```python
from build123d import *

# Parameters (mm, degrees)
BOSS_EXTRUDE1_DEPTH                               = 450
BACKSIDEHOLES_SKETCH3_R                           = 1.5875
BACKSIDEHOLES_CUT_EXTRUDE1_DEPTH                  = 3.175
RIGHTSIDEHOLES_CUT_EXTRUDE2_OUTLINE_R             = 1.5875
RIGHTSIDEHOLES_CUT_EXTRUDE2_DEPTH                 = 3.175
CSK_FOR_6_FLAT_HEAD_MACHINE_SCREW_100_D           = 3.7973
CSK_FOR_6_FLAT_HEAD_MACHINE_SCREW_100_CSINK_D     = 7.0866
CSK_FOR_6_FLAT_HEAD_MACHINE_SCREW_100_CSINK_ANGLE = 100
CSK_FOR_6_FLAT_HEAD_MACHINE_SCREW_2_D             = 3.7973
CSK_FOR_6_FLAT_HEAD_MACHINE_SCREW_2_CSINK_D       = 7.0866
CSK_FOR_6_FLAT_HEAD_MACHINE_SCREW_2_CSINK_ANGLE   = 100


# Read off the part's stored shape, not the designer's step: RightSideHoles-Cut-Extrude2
with BuildPart() as part:
    # Sketch2 → Boss-Extrude1 (new body)
    with BuildSketch(Plane(origin=(0, 0, 0), x_dir=(1, 0, 0), z_dir=(0, 1, 0))):
        Polygon((0, 31.75), (3.175, 31.75), (3.175, 3.175), (31.75, 3.175), (31.75, 0), (0, 0), align=None)
    extrude(amount=BOSS_EXTRUDE1_DEPTH)

    # BackSideHoles-Sketch3 → BackSideHoles-Cut-Extrude1 (cut)
    with BuildSketch(Plane.XY):
        with Locations((19.05, 81.1125)):
            Circle(BACKSIDEHOLES_SKETCH3_R)
        with Locations((14.2875, 87.4625)):
            Circle(BACKSIDEHOLES_SKETCH3_R)
        with Locations((23.933174186, 87.4625)):
            Circle(BACKSIDEHOLES_SKETCH3_R)
        with Locations((14.2875, 438.8875)):
            Circle(BACKSIDEHOLES_SKETCH3_R)
        with Locations((23.8125, 438.8875)):
            Circle(BACKSIDEHOLES_SKETCH3_R)
        with Locations((19.05, 426.1875)):
            Circle(BACKSIDEHOLES_SKETCH3_R)
        with Locations((14.2875, 336.74737)):
            Circle(BACKSIDEHOLES_SKETCH3_R)
        with Locations((23.8125, 336.74737)):
            Circle(BACKSIDEHOLES_SKETCH3_R)
        with Locations((19.05, 330.39737)):
            Circle(BACKSIDEHOLES_SKETCH3_R)
        with Locations((14.2875, 165)):
            Circle(BACKSIDEHOLES_SKETCH3_R)
        with Locations((14.2875, 260)):
            Circle(BACKSIDEHOLES_SKETCH3_R)
        with Locations((14.2875, 7.9375)):
            Circle(BACKSIDEHOLES_SKETCH3_R)
        with Locations((23.8125, 7.9375)):
            Circle(BACKSIDEHOLES_SKETCH3_R)
        with Locations((14.2875, 355)):
            Circle(BACKSIDEHOLES_SKETCH3_R)
    extrude(amount=-BACKSIDEHOLES_CUT_EXTRUDE1_DEPTH, mode=Mode.SUBTRACT)

    # RightSideHoles-Cut-Extrude2 outline → RightSideHoles-Cut-Extrude2 (cut)
    with BuildSketch(Plane.YZ):
        with Locations((81.1125, -23.8125)):
            Circle(RIGHTSIDEHOLES_CUT_EXTRUDE2_OUTLINE_R)
        with Locations((306.32237, -23.8125)):
            Circle(RIGHTSIDEHOLES_CUT_EXTRUDE2_OUTLINE_R)
        with Locations((341.24737, -14.2875)):
            Circle(RIGHTSIDEHOLES_CUT_EXTRUDE2_OUTLINE_R)
        with Locations((341.24737, -23.8125)):
            Circle(RIGHTSIDEHOLES_CUT_EXTRUDE2_OUTLINE_R)
        with Locations((165, -14.2875)):
            Circle(RIGHTSIDEHOLES_CUT_EXTRUDE2_OUTLINE_R)
        with Locations((306.32237, -14.2875)):
            Circle(RIGHTSIDEHOLES_CUT_EXTRUDE2_OUTLINE_R)
        with Locations((260, -14.2875)):
            Circle(RIGHTSIDEHOLES_CUT_EXTRUDE2_OUTLINE_R)
        with Locations((81.1125, -14.2875)):
            Circle(RIGHTSIDEHOLES_CUT_EXTRUDE2_OUTLINE_R)
        with Locations((87.4625, -19.05)):
            Circle(RIGHTSIDEHOLES_CUT_EXTRUDE2_OUTLINE_R)
        with Locations((355, -14.2875)):
            Circle(RIGHTSIDEHOLES_CUT_EXTRUDE2_OUTLINE_R)
        with Locations((438.8875, -19.05)):
            Circle(RIGHTSIDEHOLES_CUT_EXTRUDE2_OUTLINE_R)
        with Locations((426.1875, -14.2875)):
            Circle(RIGHTSIDEHOLES_CUT_EXTRUDE2_OUTLINE_R)
        with Locations((426.1875, -23.8125)):
            Circle(RIGHTSIDEHOLES_CUT_EXTRUDE2_OUTLINE_R)
        with Locations((7.9375, -23.8125)):
            Circle(RIGHTSIDEHOLES_CUT_EXTRUDE2_OUTLINE_R)
        with Locations((7.9375, -14.2875)):
            Circle(RIGHTSIDEHOLES_CUT_EXTRUDE2_OUTLINE_R)
    extrude(amount=RIGHTSIDEHOLES_CUT_EXTRUDE2_DEPTH, mode=Mode.SUBTRACT)

    # CSK for _6 Flat Head Machine Screw _100 (through all)
    with Locations(Plane.ZY):
        with Locations((-23.8125, 81.1125), (-19.05, 87.4625), (-14.2875, 81.1125), (-23.8125, 341.24737), (-14.2875, 341.24737), (-23.8125, 306.32237), (-14.2875, 306.32237), (-23.8125, 426.1875), (-14.2875, 426.1875), (-19.05, 438.8875)):
            CounterSinkHole(CSK_FOR_6_FLAT_HEAD_MACHINE_SCREW_100_D / 2, CSK_FOR_6_FLAT_HEAD_MACHINE_SCREW_100_CSINK_D / 2, counter_sink_angle=CSK_FOR_6_FLAT_HEAD_MACHINE_SCREW_100_CSINK_ANGLE)

    # CSK for _6 Flat Head Machine Screw _ 2 (through all)
    with Locations(Plane.XY):
        with Locations((14.2875, 336.74737), (23.8125, 336.74737), (19.05, 330.39737), (19.05, 426.1875), (23.8125, 438.8875), (14.2875, 438.8875), (14.2875, 87.4625), (23.933174186, 87.4625), (19.05, 81.1125)):
            CounterSinkHole(CSK_FOR_6_FLAT_HEAD_MACHINE_SCREW_2_D / 2, CSK_FOR_6_FLAT_HEAD_MACHINE_SCREW_2_CSINK_D / 2, counter_sink_angle=CSK_FOR_6_FLAT_HEAD_MACHINE_SCREW_2_CSINK_ANGLE)


solid = part.part
```
Geometry check sheet. Reference: the model listing, model coordinates, mm. A direction names the side the tool comes from. Coordinates: 2 decimals unless noted, no trailing zeros. Order: outer loops, then holes, each group sorted by start corner. A loop starts at its lowest first (then second) coordinate and runs counter-clockwise, first axis right, second up.
Q1. Depth check by flat-ended pin: pin 1 Ø4.5 at (x, y) = (19.05, 81.11) entering from +Z; pin 2 Ø2.5 at (y, z) = (355, -14.29) entering from +X; pin 3 Ø5 at (x, y) = (14, 363.5) entering from -Z (3 decimals); pin 4 Ø5 at (y, z) = (81.11, -14.29) entering from +X (3 decimals). Enter the tip coordinate at first touch or a pass-through.
Reply:
pin 1: stops at z = -1.08
pin 2: passes through
pin 3: stops at z = -3.175
pin 4: stops at x = 3.175
Q2. Thickness scan on probe 1 along Y at (x, z) = (23, -2.5); probe 2 along Z at (x, y) = (29, 227) (3 decimals); probe 3 along X at (y, z) = (105, -28) (3 decimals). Record the ranges inside material, lowest first.
Reply:
probe 1: y = 0 to 6.57, 9.3 to 85.81, 89.12 to 335.03, 338.46 to 437.17, 440.6 to 450
probe 2: z = -3.175 to 0
probe 3: x = 0 to 3.175
Q3. Tool access check on faces 1 (the face through (17, 222, -3.175)), 2 (the face through (12, 88, -1)). Record the directions out of +Z, -Z, +X, -X, +Y, -Y that give a thin tool (end or side, any length) a straight path to the whole face; none if there is none.
Reply:
face 1: -Z, +X, +Y, -Y
face 2: +Z
Q4. Sectioned sample at A-A on y = 104. Record the cut outline in (x, z) (3 decimals), and give its area (3 significant figures).
Reply:
outline: (0, -31.75) - (3.175, -31.75) - (3.175, -3.175) - (31.75, -3.175) - (31.75, 0) - (0, 0) - close
area: 192 mm2
Q5. Sectioned sample at B-B on x = 7. Record the cut outline in (y, z) (3 decimals), and give its area (3 significant figures).
Reply:
outline: (0, -3.175) - (450, -3.175) - (450, 0) - (0, 0) - close
area: 1,430 mm2
